from build123d import *

# Parameters (mm, degrees)
SKETCH1_R           = 2.15
BOSS_EXTRUDE1_DEPTH = 4.45
FILLET1_R           = 3


with BuildPart() as part:
    # Sketch1 → Boss-Extrude1 (new body)
    with BuildSketch(Plane(origin=(7.87040158, 0, -4.543978471), x_dir=(0.5, 0, 0.866025404), z_dir=(-0.866025404, 0, 0.5))):
        Polygon((53.851280609, 136.798849573), (28.020561976, 136.798849573), (25.605878822, 136.798849573), (13.788638888, 118.055853922), (68.083203696, 118.055853922), (56.265963763, 136.798849573), align=None)
        with Locations((21.039254626, 122.055853922)):
            Circle(SKETCH1_R, mode=Mode.SUBTRACT)
        Polygon((53.501781192, 121.427351747), (28.370061392, 121.427351747), (35.935921292, 133.427351747), (45.935921292, 133.427351747), align=None, mode=Mode.SUBTRACT)
        with BuildLine():
            ThreePointArc((28.307564738, 134.891096687), (29.498811561, 134.132697376), (29.962587959, 132.798849573))
            ThreePointArc((29.962587959, 132.798849573), (28.449874626, 130.745470479), (26.040387304, 131.581555509))
            Line((26.040387304, 131.581555509), (25.535036631, 130.843863418))
            Line((25.535036631, 130.843863418), (25.213105243, 131.064400205))
            ThreePointArc((25.213105243, 131.064400205), (24.994059417, 131.449211896), (24.831600224, 131.861119802))
            Line((24.831600224, 131.861119802), (25.010769387, 134.182842957))
            ThreePointArc((25.010769387, 134.182842957), (25.234503174, 134.564948053), (25.509996288, 134.911595794))
            Line((25.509996288, 134.911595794), (27.610252102, 135.917292326))
            ThreePointArc((27.610252102, 135.917292326), (28.053031716, 135.91458573), (28.490984023, 135.849325565))
            Line((28.490984023, 135.849325565), (28.812915411, 135.628788778))
            Line((28.812915411, 135.628788778), (28.307564738, 134.891096687))
        make_face(mode=Mode.SUBTRACT)
        with Locations((54.059254626, 132.798849573)):
            Circle(SKETCH1_R, mode=Mode.SUBTRACT)
        with Locations((60.832587959, 122.055853922)):
            Circle(SKETCH1_R, mode=Mode.SUBTRACT)
        Polygon((28.020561976, 136.798849573), (28.577056843, 200.566845224), (53.294785741, 200.566845224), (53.851280609, 136.798849573), (56.265963763, 136.798849573), (55.69201516, 202.566845224), (26.179827424, 202.566845224), (25.605878822, 136.798849573), align=None)
        with BuildLine():
            ThreePointArc((26.040387304, 131.581555509), (26.038865627, 134.013925327), (28.307564738, 134.891096687))
            Line((28.307564738, 134.891096687), (28.812915411, 135.628788778))
            Line((28.812915411, 135.628788778), (28.490984023, 135.849325565))
            ThreePointArc((28.490984023, 135.849325565), (28.053031716, 135.91458573), (27.610252102, 135.917292326))
            Line((27.610252102, 135.917292326), (25.509996288, 134.911595794))
            ThreePointArc((25.509996288, 134.911595794), (25.234503174, 134.564948053), (25.010769387, 134.182842957))
            Line((25.010769387, 134.182842957), (24.831600224, 131.861119802))
            ThreePointArc((24.831600224, 131.861119802), (24.994059417, 131.449211896), (25.213105243, 131.064400205))
            Line((25.213105243, 131.064400205), (25.535036631, 130.843863418))
            Line((25.535036631, 130.843863418), (26.040387304, 131.581555509))
        make_face()
    extrude(amount=BOSS_EXTRUDE1_DEPTH)

    # Fillet1
    fillet1_edges = [part.edges().sort_by_distance(p)[0] for p in [
        (12.8378145, 118.055853922, 8.50983309),
        (18.746434467, 136.798849573, 18.743863075),
        (19.033408769, 202.566845224, 19.240917146),
        (33.789502636, 202.566845224, 44.799221446),
        (34.076476938, 136.798849573, 45.296275517),
        (39.985096905, 118.055853922, 55.530305501),
    ]]
    fillet(fillet1_edges, radius=FILLET1_R)


solid = part.part
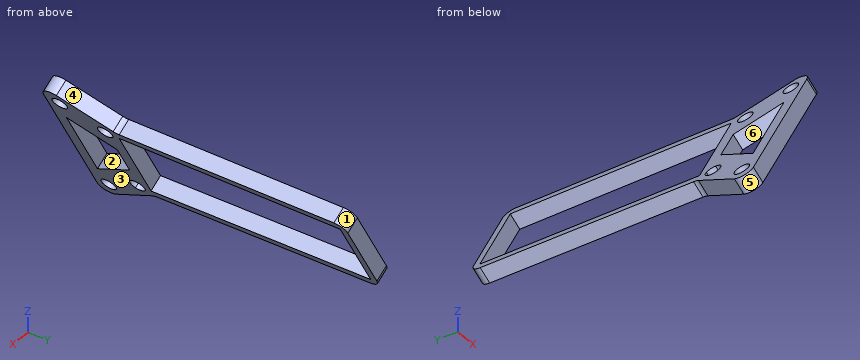
For this review, take the finished solid that the model builds, in its own axes (mm). Face numbers are marked on the shaded views. A direction names the side the tool comes from. Give positions to 0.01 mm unless a question says otherwise; leave off trailing zeros. Order: outer loops, then holes, each group sorted by start corner. A loop starts at its lowest first (then second) coordinate and runs counter-clockwise, first axis right, second up. Notation, with made-up numbers: M 7.25,26 L 29.25,26 A10 cw 29.25,43 Z; hole C -13,76 d5. An arc over 180 degrees is marked long. Answer in a Markdown table with one row per item. Add a question column.
(1) Mouldability with a two-part tool opening along Y and no side actions: class the marked faces 3, 4, 5 and 6 as +Y half, -Y half, draft (parallel to the pull), parting line (faces both ways), or undercut.
(2) Consider section A-A on y = 160. State the section outline as (x, z) points.
(3) For the marked faces 1 and 2, list the 3-axis set-ups (+Z, -Z, +X, -X, +Y, -Y) from which the entire face can be reached by the end or side of a thin tool; tool diameter is ignored.
(4) Wall thickness on probe 1 along Y at (x, z) = (23, 29.5); probe 2 along Y at (x, z) = (30, 37); probe 3 along Z at (x, y) = (19.75, 196.5): over which ranges is each line inside the solid? List them lowest first. Write a range as [from, to].
(5) Consider section B-B on z = 34. State the section outline as (x, y) points, and give its area (3 significant figures).
(6) For pin 1 (8 mm diameter, centred on x = 34, z = 48.5, fed in from +Y); pin 2 (3 mm diameter, centred on x = 23.5, y = 181, fed in from -Z); pin 3 (10 mm diameter, centred on y = 191.5, z = 48, fed in from -X), all flat-tipped, find the tip position at first contact; note any pin that passes through.
Evaluation:
| question | item | result |
|---|---|---|
| 1 | face 3 | draft |
| 1 | face 4 | +Y half |
| 1 | face 5 | parting line |
| 1 | face 6 | undercut |
| 2 | outline | M 16.92,20.03 L 20.77,17.81 L 21.98,19.9 L 18.13,22.12 Z; M 30.84,44.14 L 34.69,41.92 L 35.9,44.01 L 32.05,46.23 Z |
| 3 | face 1 | +Z, +X, +Y |
| 3 | face 2 | +Z, +X |
| 4 | probe 1 | y = [118.06, 121.43], [133.43, 136.8], [200.57, 202.57] |
| 4 | probe 2 | y = [118.06, 121.43], [131.67, 136.8], [200.57, 202.57] |
| 4 | probe 3 | z = [18.77, 21.55] |
| 5 | outline | M 24.99,118.06 L 30.12,118.06 L 30.12,121.43 L 24.99,121.43 Z; M 24.99,133.43 L 30.12,133.43 L 30.12,136.8 L 24.99,136.8 Z; M 24.99,200.57 L 30.12,200.57 L 30.12,202.57 L 24.99,202.57 Z |
| 5 | area | 44.9 mm^2 |
| 6 | pin 1 | stops at y = 201.51 |
| 6 | pin 2 | stops at z = 19.93 |
| 6 | pin 3 | stops at x = 30.69 |
